Check sheet for the drawn part. Datum: minimum x, y, z corner. Units: mm. A direction names the side the tool comes from. Give positions to 0.01 mm unless a question says otherwise; leave off trailing zeros. Write each loop counter-clockwise with the first axis right and the second up, starting at its lowest first coordinate (ties: lowest second). Pieces come first, ordered by that corner, then holes. Notation, with made-up numbers: (57.5, 8) - (103.5, 8) arc R24 ccw to (103.5, 40) - close; hole circle Ø5 at (14.25, 73.25). An arc over 180 degrees is marked (long way). Answer as a JSON object with one key per item and string values. Group by question number.
Item 1: Sectioned sample at C-C, the plane x = 34.5. Record the boundary of the cut face in (y, z).
Item 2: Draft check along X on the marked faces 3, 4 and 5. Enter one of: +X half, -X half, draft (parallel to the pull), parting line (faces both ways), or undercut.
Item 3: Go/stop test with a flat-tipped pin: pin 1 (11.5 mm diameter, centred on x = 27, y = 24.5, fed in from +Z). Record where the tip stops, or that it passes through.
Item 4: Sectioned sample at B-B, the plane y = 9.5. Record the boundary of the cut face in (x, z).
Item 5: Sectioned sample at A-A, the plane z = 4. Record the boundary of the cut face in (x, y).
Item 6: Tool access check on the marked faces 1 and 2. Record the directions out of +Z, -Z, +X, -X, +Y, -Y that give a thin tool (end or side, any length) a straight path to the whole face; none if there is none.
Item 7: Scan lines: line 1 along X through (y, z) = (20, 5.25); line 2 along Y through (x, z) = (40.5, 4.25); line 3 along Z through (x, y) = (5, 20). Record each from-to range of solid material in increasing order. Write a range as [from, to].
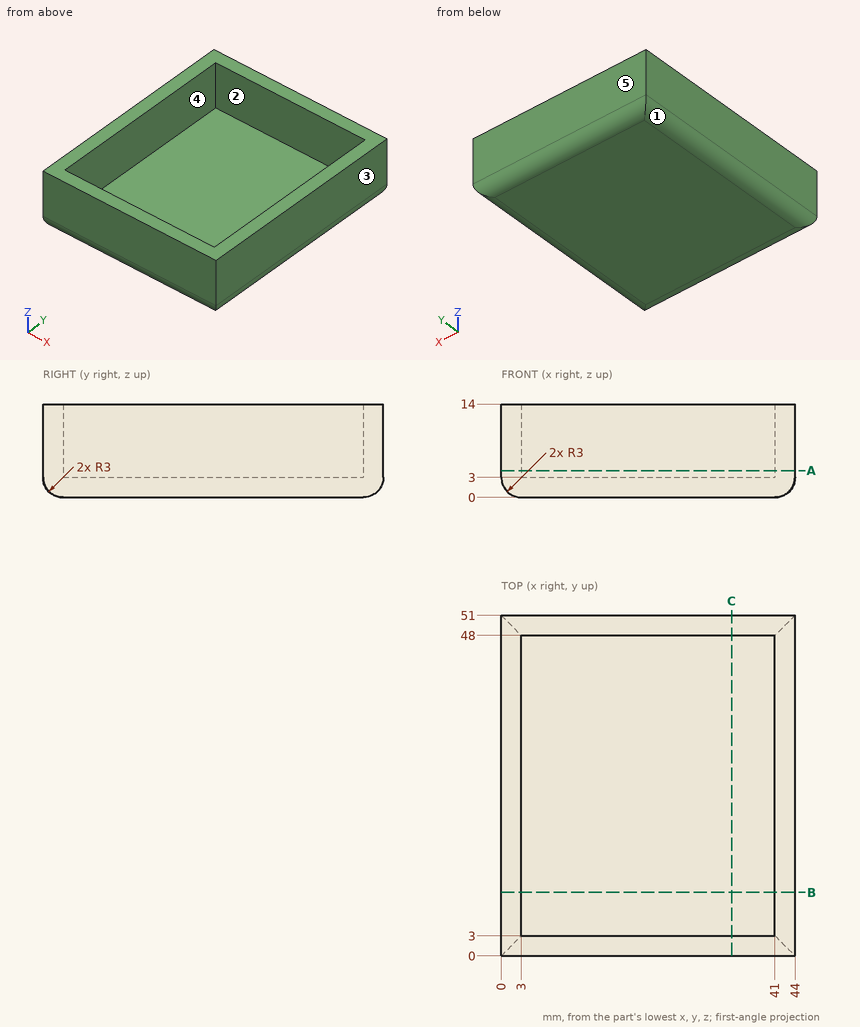
Geometry check:
{
 "1": {"outline": "(0, 3) arc R3 ccw to (3, 0) - (48, 0) arc R3 ccw to (51, 3) - (51, 14) - (48, 14) - (48, 3) - (3, 3) - (3, 14) - (0, 14) - close"},
 "2": {"face 3": "+X half", "face 4": "undercut", "face 5": "draft"},
 "3": {"pin 1": "z = 3"},
 "4": {"outline": "(0, 3) arc R3 ccw to (3, 0) - (41, 0) arc R3 ccw to (44, 3) - (44, 14) - (41, 14) - (41, 3) - (3, 3) - (3, 14) - (0, 14) - close"},
 "5": {"outline": "(0, 0) - (44, 0) - (44, 51) - (0, 51) - close; hole (3, 3) - (41, 3) - (41, 48) - (3, 48) - close"},
 "6": {"face 1": "-Z, -X, +Y, -Y", "face 2": "+Z"},
 "7": {"line 1": "[0, 3], [41, 44]", "line 2": "[0, 3], [48, 51]", "line 3": "[0, 3]"}
}
